Could you check a few things on this model? Use its own coordinates, in mm. Face numbers are marked on the shaded views. Coordinates: 2 decimals unless noted, no trailing zeros. Loops run counter-clockwise (first coordinate to the right, second up) from the corner with the lowest first, then second, coordinate; pieces in that order, holes last.
Autodesk Inventor part; units mm, degrees
ref_plane "YZ Plane" through (0, 0, 0) normal (1, 0, 0) x (0, 1, 0)
ref_plane "XZ Plane" through (0, 0, 0) normal (0, 1, 0) x (-1, 0, 0)
ref_plane "XY Plane" through (0, 0, 0) normal (0, 0, 1) x (1, 0, 0)
sketch "Sketch1" plane through (0, 0, 0) normal (0, 0, 1) x (1, 0, 0)
  arc A0 (77.1345, 91.9253) -> (-120, 0) centre (0, 0) ccw
  arc A1 (57.8509, 68.944) -> (-90, 0) centre (0, 0) ccw
  line L0 (-120, 0) -> (-90, 0) construction
  line L1 (0, 0) -> (77.1345, 91.9253) construction
  line L2 (57.8509, 68.944) -> (77.1345, 91.9253) construction
  arc A2 (-120, 0) -> (-90, 0) centre (-105, 0) ccw
  arc A3 (57.8509, 68.944) -> (77.1345, 91.9253) centre (67.4927, 80.4347) ccw
  dimension "d0" = 240
  dimension "d1" = 30
  dimension "d2" = 130
extrude "Extrusion2" add sketch "Sketch1" along normal blind 1
sketch "Sketch2" plane through (0, 0, 1) normal (0, 0, 1) x (1, 0, 0)
  arc A0 (77.1345, 91.9253) -> (-120, 0) centre (0, 0) ccw
  arc A1 (-120, 0) -> (-90, 0) centre (-105, 0) ccw
  circle A2 centre (-110, -8) radius 5
  arc A3 (57.8509, 68.944) -> (-90, 0) centre (0, 0) ccw
  arc A4 (57.8509, 68.944) -> (77.1345, 91.9253) centre (67.4927, 80.4347) ccw
  line L0 (57.8509, 68.944) -> (77.1345, 91.9253) construction
  circle A5 centre (69.4211, 82.7328) radius 5
  line L1 (-120, 0) -> (-90, 0) construction
  line L2 (-120, 0) -> (-120, 14.4317) construction
  line L3 (77.1345, 91.9253) -> (63.1812, 103.6336) construction
  dimension "d10" = 10
  dimension "d12" = 10
  dimension "d20" = 10
  dimension "d21" = 8
  dimension "d22" = 90
  dimension "d23" = 12
  dimension "d24" = 0
  dimension "d25" = 82.7328
  dimension "d26" = 189.4211
extrude "Extrusion3" cut sketch "Sketch2" against normal through all contours A2 | A5
sketch "Sketch3" plane through (0, 0, 1) normal (0, 0, 1) x (1, 0, 0)
  arc A0 (-120, 0) -> (-90, 0) centre (-105, 0) ccw
  line L0 (-120, 0) -> (-90, 0) construction
  line L1 (-120, 0) -> (-109.6077, -6)
  line L2 (-109.6077, -6) -> (-91.2523, -6)
  arc A1 (-120, 0) -> (-90, 0) centre (-105, 0) ccw
  point P0 (0, 0)
  dimension "d16" = 30
  dimension "d17" = 6
extrude "Extrusion4" [suppressed]
equation "\"d0\" = diametro_max"
equation "\"d1\" = ancho_disco"
equation "\"d2\" = angulo_alabe"
equation "\"d10\" = diametro_pin"
equation "\"d12\" = d10"
equation "\"d20\" = desfase_a_pin_inferior"
equation "\"d21\" = desfase_b_pin_inferior"
equation "\"d23\" = desfase_a_pin_superior"
equation "\"angulo_alabe\" = 130deg"
equation "\"ancho_disco\" = 30"
equation "\"diametro_max\" = 240"
equation "\"diametro_tubo\" = 232"
equation "\"desfase_pin_superior\" = 12"
equation "\"desfase_b_pin_inferior\" = 8"
equation "\"desfase_a_pin_inferior\" = 10"
equation "\"desfase_b_pin_superior\" = 0"
equation "\"desfase_a_pin_superior\" = 12"
equation "\"diametro_pin\" = 10"
equation "\"diametro_max_soporte\" = 248"
properties part number "alabes"
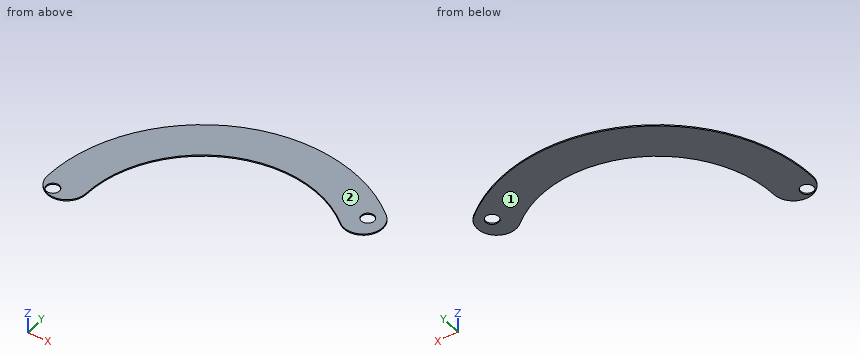
1) Imagine slicing it at B-B on x = -110. List the corners of the cut face in (y, z) for me, plus the area to 3 significant figures.
2) Imagine slicing it at C-C on z = 0.55. List the corners of the cut face in (x, y) for me.
3) Imagine slicing it at A-A on y = -8. List the corners of the cut face in (x, z) for me.
4) We'd pull the mould along Z, two halves only. Please class the marked faces 1 and 2: released by +Z, released by -Z, zero draft, split by the parting line, or undercut.
5) Will this pin go through, and if not, where does the flat tip stop? pin 1 (9 mm diameter, centred on x = -110, y = -8, fed in from +Z).
6) Imagine slicing it at D-D on x = 15.5. List the corners of the cut face in (y, z) for me, plus the area to 3 significant figures.
7) If I drill on L1, parallel to Y at x = -110, z = 0.65; L2, parallel to Y at x = 2.5, z = 0.45; L3, parallel to X at y = -7.5, z = 0.5, over which ranges is the centre line in solid material (lowest first)?
Solved:
1. outline: (-14.14, 0) - (-13, 0) - (-13, 1) - (-14.14, 1) - close; (-3, 0) - (47.96, 0) - (47.96, 1) - (-3, 1) - close
1. area: 52.1 mm2
2. outline: (-120, 0) arc R15 ccw to (-90, 0) arc R90 cw to (57.85, 68.94) arc R15 ccw to (77.13, 91.93) arc R120 ccw to start; hole circle Ø10 at (-110, -8); hole circle Ø10 at (69.42, 82.73)
3. outline: (-117.69, 0) - (-115, 0) - (-115, 1) - (-117.69, 1) - close; (-105, 0) - (-92.31, 0) - (-92.31, 1) - (-105, 1) - close
4. face 1: released by -Z
4. face 2: released by +Z
5. pin 1: passes through
6. outline: (88.66, 0) - (118.99, 0) - (118.99, 1) - (88.66, 1) - close
6. area: 30.3 mm2
7. L1: y = -14.14 to -13, -3 to 47.96
7. L2: y = 89.97 to 119.97
7. L3: x = -117.99 to -114.97, -105.03 to -92.01
